from build123d import *

# Parameters (mm, degrees)
SKETCH1_W           = 800
SKETCH1_H           = 800
BOSS_EXTRUDE1_DEPTH = 450
SHELL1_T            = -5
SKETCH2_W           = 790
SKETCH2_H           = 395
BOSS_EXTRUDE2_DEPTH = 300
CUT_EXTRUDE1_START  = -5
SKETCH3_R           = 40
CUT_EXTRUDE1_DEPTH  = 790
SKETCH4_W           = 50
SKETCH4_H           = 50
BOSS_EXTRUDE3_DEPTH = 130


with BuildPart() as part:
    # Sketch1 → Boss-Extrude1 (new body)
    with BuildSketch(Plane(origin=(0, 0, 0), x_dir=(1, 0, 0), z_dir=(0, 1, 0))):
        with Locations((400, -400)):
            Rectangle(SKETCH1_W, SKETCH1_H)
    extrude(amount=BOSS_EXTRUDE1_DEPTH)

    # Shell1
    shell1_openings = [part.faces().sort_by_distance(p)[0] for p in [
        (400, 450, 400),
    ]]
    offset(amount=SHELL1_T, openings=shell1_openings, kind=Kind.INTERSECTION)

    # Sketch2 → Boss-Extrude2 (add)
    with BuildSketch(Plane(origin=(0, 5, 0), x_dir=(1, 0, 0), z_dir=(0, 1, 0))):
        with Locations((400, -597.5)):
            Rectangle(SKETCH2_W, SKETCH2_H)
    extrude(amount=BOSS_EXTRUDE2_DEPTH)

    # Sketch3 → Cut-Extrude1 (cut)
    with BuildSketch(Plane(origin=(800, 0, 0), x_dir=(0, 0, -1), z_dir=(1, 0, 0)).offset(CUT_EXTRUDE1_START)):
        with Locations((-600, 305)):
            Circle(SKETCH3_R)
    extrude(amount=-CUT_EXTRUDE1_DEPTH, mode=Mode.SUBTRACT)

    # Sketch4 → Boss-Extrude3 (add)
    with BuildSketch(Plane.XZ):
        with Locations((25, 775)):
            Rectangle(SKETCH4_W, SKETCH4_H)
        with Locations((400, 775)):
            Rectangle(SKETCH4_W, SKETCH4_H)
        with Locations((775, 775)):
            Rectangle(SKETCH4_W, SKETCH4_H)
        with Locations((400, 400)):
            Rectangle(SKETCH4_W, SKETCH4_H)
        with Locations((775, 400)):
            Rectangle(SKETCH4_W, SKETCH4_H)
        with Locations((400, 25)):
            Rectangle(SKETCH4_W, SKETCH4_H)
        with Locations((775, 25)):
            Rectangle(SKETCH4_W, SKETCH4_H)
        with Locations((25, 400)):
            Rectangle(SKETCH4_W, SKETCH4_H)
        with Locations((25, 25)):
            Rectangle(SKETCH4_W, SKETCH4_H)
    extrude(amount=BOSS_EXTRUDE3_DEPTH)


solid = part.part
Could you check a few things on this model? Use its own coordinates, in mm. A direction names the side the tool comes from. Give positions to 0.01 mm unless a question says otherwise; leave off trailing zeros. Order: outer loops, then holes, each group sorted by start corner. A loop starts at its lowest first (then second) coordinate and runs counter-clockwise, first axis right, second up. Notation, with made-up numbers: M -15,32.5 L -5,32.5 A28 ccw -5,58.5 Z; hole C 13.25,-12.75 d9. An arc over 180 degrees is marked long. One line per question, with ' | ' between items.
1. If I drill on line 1 (Z direction, x = 755.5, y = 190); line 2 (Z direction, x = 378, y = 337), over which ranges is the centre line in solid material (lowest first)?
Results:
line 1: 0 to 5, 400 to 800 | line 2: 0 to 5, 795 to 800
2. For faces 1 (the face through (775, -130, 400)), 2 (the face through (394, 305, 716)), 3 (the face through (394, 229, 800)), 4 (the face through (375, -64, 775)), 5 (the face through (775, -64, 425)), which set-ups out of +Z, -Z, +X, -X, +Y, -Y let a thin tool reach every point of the face, with its end or its side?
Results:
face 1: +Z, -Z, +X, -X, -Y | face 2: +Y | face 3: +Z, +X, -X, +Y, -Y | face 4: +Z, -Z, -Y | face 5: +X, -X, -Y
3. I want a section at C-C (y = 39). List the corners of the cut face in (x, z) for me, and give its area (3 significant figures).
Results:
outline: M 0,0 L 800,0 L 800,800 L 0,800 Z; hole M 5,5 L 795,5 L 795,400 L 5,400 Z | area: 328,000 mm²
4. I want a section at D-D (z = 600). List the corners of the cut face in (x, y) for me, and give its area (3 significant figures).
Results:
outline: M 0,0 L 800,0 L 800,450 L 795,450 L 795,265 L 5,265 L 5,450 L 0,450 Z | area: 214,000 mm²
5. I want a section at A-A (x = 497.5). List the corners of the cut face in (y, z) for me, and give its area (3 significant figures).
Results:
outline: M 0,0 L 450,0 L 450,5 L 5,5 L 5,400 L 305,400 L 305,560 A40 cw 305,640 L 305,795 L 450,795 L 450,800 L 0,800 Z | area: 124,000 mm²
6. I want a section at B-B (z = 138). List the corners of the cut face in (x, y) for me.
Results:
outline: M 0,0 L 800,0 L 800,450 L 795,450 L 795,5 L 5,5 L 5,450 L 0,450 Z
7. I'm going to push flat-ended pins straight in: pin 1 (10 mm diameter, centred on x = 441.5, z = 261, fed in from -Y); pin 2 (4 mm diameter, centred on x = 413, y = 42.5, fed in from -Z); pin 3 (5 mm diameter, centred on x = 250.5, z = 434.5, fed in from +Y). Where does each tip first touch, or does it pass through?
Results:
pin 1: y = 0 | pin 2: z = 0 | pin 3: y = 305
8. We'd pull the mould along X, two halves only. Please class faces 6 (the face through (25, -64, 750)), 7 (the face through (750, -64, 25)), 8 (the face through (0, 229, 394)): +X half, -X half, draft (parallel to the pull), parting line (faces both ways), or undercut.
Results:
face 6: draft | face 7: undercut | face 8: -X half
